Design review of the part built by this model. Coordinates are the model's own, in mm. Face numbers are marked on the shaded views. A direction names the side the tool comes from. Coordinates: 2 decimals unless noted, no trailing zeros. Loops run counter-clockwise (first coordinate to the right, second up) from the corner with the lowest first, then second, coordinate; pieces in that order, holes last.
Q1. Add section B-B on z = 23.25. Give the boundary of the cut face in (x, y).
Q2. Wall thickness on probe 1 along Y at (x, z) = (0, 7.25); probe 2 along Y at (x, z) = (15, 19.75); probe 3 along Z at (x, y) = (-10, -25): over which ranges is each line inside the solid? List them lowest first.
Q3. Add section A-A on y = 0. Give the boundary of the cut face in (x, z), and give its area (3 significant figures).
Q4. Machinability: for the marked faces 1, 2 and 3, which of the approach directions +Z, -Z, +X, -X, +Y, -Y give a long, thin tool a straight path to every point of the face, cutting with its end or side? Answer none if there is none.
Q5. Add section D-D on y = -14.5. Give the boundary of the cut face in (x, z), and give its area (3 significant figures).
Q6. For P1, Ø10, axis at y = -6, z = 5.5, coming from the -X side; P2, Ø3, axis at x = -25.11, y = -14.5, coming from the +Z side; P3, Ø3, axis at y = 14, z = 16.5, coming from the -X side; P4, Ø8, axis at y = 16, z = 15, coming from the +X side, all flat-tipped, find the tip position at first contact; note any pin that passes through.
Q7. Add section C-C on x = 0. Give the boundary of the cut face in (y, z).
Q8. Draft analysis for pull direction Y (two halves, no side actions). For the marked faces 4, 5 and 6, state which applies: released by +Y, released by -Y, zero draft, split by the parting line, or undercut.
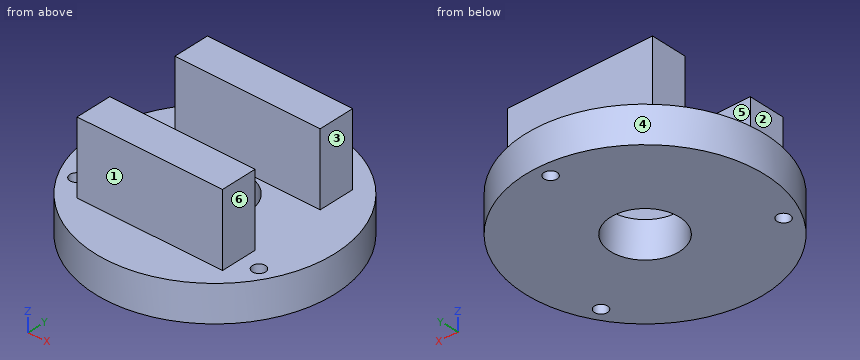
```python
from build123d import *

# Parameters (mm, degrees)
SKETCH_1_R      = 33
SKETCH_1_R_2    = 1.8
SKETCH_1_R_3    = 9.5
EXTRUDE_1_DEPTH = 10
SKETCH_2_W      = 40
SKETCH_2_H      = 10
EXTRUDE_2_DEPTH = 20


with BuildPart() as part:
    # 草图1 → 凸台-拉伸1 (new body)
    with BuildSketch(Plane.XY):
        Circle(SKETCH_1_R)
        with Locations((0, 29)):
            Circle(SKETCH_1_R_2, mode=Mode.SUBTRACT)
        with Locations((25.11473671, -14.5)):
            Circle(SKETCH_1_R_2, mode=Mode.SUBTRACT)
        with Locations((-25.11473671, -14.5)):
            Circle(SKETCH_1_R_2, mode=Mode.SUBTRACT)
        Circle(SKETCH_1_R_3, mode=Mode.SUBTRACT)
    extrude(amount=EXTRUDE_1_DEPTH)

    # 草图2 → 凸台-拉伸2 (add)
    with BuildSketch(Plane.XY.offset(10)):
        with Locations((0, 15)):
            Rectangle(SKETCH_2_W, SKETCH_2_H)
        with Locations((0, -15)):
            Rectangle(SKETCH_2_W, SKETCH_2_H)
    extrude(amount=EXTRUDE_2_DEPTH)


solid = part.part
```
Entries:
1. outline: (-20, -20) - (20, -20) - (20, -10) - (-20, -10) - close; (-20, 10) - (20, 10) - (20, 20) - (-20, 20) - close
2. probe 1: y = -33 to -9.5, 9.5 to 27.2, 30.8 to 33
2. probe 2: y = -20 to -10, 10 to 20
2. probe 3: z = 0 to 10
3. outline: (-33, 0) - (-9.5, 0) - (-9.5, 10) - (-33, 10) - close; (9.5, 0) - (33, 0) - (33, 10) - (9.5, 10) - close
3. area: 470 mm2
4. face 1: +Z, +X, -X, -Y
4. face 2: +Z, -X, +Y, -Y
4. face 3: +Z, +X, +Y, -Y
5. outline: (-29.64, 0) - (-26.91, 0) - (-26.91, 10) - (-29.64, 10) - close; (-23.31, 0) - (23.31, 0) - (23.31, 10) - (20, 10) - (20, 30) - (-20, 30) - (-20, 10) - (-23.31, 10) - close; (26.91, 0) - (29.64, 0) - (29.64, 10) - (26.91, 10) - close
5. area: 1,320 mm2
6. P1: stops at x = -32.98
6. P2: passes through
6. P3: stops at x = -20
6. P4: stops at x = 20
7. outline: (-33, 0) - (-9.5, 0) - (-9.5, 10) - (-10, 10) - (-10, 30) - (-20, 30) - (-20, 10) - (-33, 10) - close; (9.5, 0) - (27.2, 0) - (27.2, 10) - (20, 10) - (20, 30) - (10, 30) - (10, 10) - (9.5, 10) - close; (30.8, 0) - (33, 0) - (33, 10) - (30.8, 10) - close
8. face 4: split by the parting line
8. face 5: undercut
8. face 6: zero draft
